from build123d import *

# Parameters (mm, degrees)
SKETCH1_W           = 315
SKETCH1_H           = 12.7
SKETCH1_W_2         = 50
BOSS_EXTRUDE1_DEPTH = 12.7
SKETCH2_R           = 3.75
CUT_EXTRUDE1_DEPTH  = 318.513983944


with BuildPart() as part:
    # Sketch1 → Boss-Extrude1 (new body)
    with BuildSketch(Plane(origin=(0, 0, 0), x_dir=(0, 0, -1), z_dir=(1, 0, 0))):
        with Locations((157.5, 6.35)):
            Rectangle(SKETCH1_W, SKETCH1_H)
        Polygon((15, 0), (0, 0), (0, -37.8), (15, -37.8), (15, -25.1), align=None)
        with Locations((40, -31.45)):
            Rectangle(SKETCH1_W_2, SKETCH1_H)
    extrude(amount=BOSS_EXTRUDE1_DEPTH)

    # Sketch2 → Cut-Extrude1 (cut, through all)
    with BuildSketch(Plane(origin=(12.7, 0, 0), x_dir=(0, 0, -1), z_dir=(1, 0, 0))):
        with Locations((7.5, 6.35)):
            Circle(SKETCH2_R)
        with Locations((207.5, 6.35)):
            Circle(SKETCH2_R)
    extrude(amount=-CUT_EXTRUDE1_DEPTH, mode=Mode.SUBTRACT)


solid = part.part
Read the model definition and answer for the solid it produces. Units are mm, in the model's axes. A direction names the side the tool comes from. Round coordinates to 2 decimals unless told otherwise and drop trailing zeros. Loops run counter-clockwise (first coordinate to the right, second up) from the corner with the lowest first, then second, coordinate; pieces in that order, holes last.
Q1. Section A-A on z = -207.5 is taken. Write down the section's boundary in (x, y), and give its area (3 significant figures).
Q2. Determine the mould class of faces 4 (the face through (6.439, 10.068, -7.012)), 5 (the face through (0, 1, -133)), 6 (the face through (6, 6, -315)) for opening direction Z: released by +Z, released by -Z, zero draft, split by the parting line, or undercut.
Q3. Section D-D on z = -7.5 is taken. Write down the section's boundary in (x, y).
Q4. Section B-B on x = 9 is taken. Write down the section's boundary in (y, z), and give its area (3 significant figures).
Q5. Which of the six approach directions +Z, -Z, +X, -X, +Y, -Y give full straight-line access (tool end or side, diameter ignored) to faces 1 (the face through (6, -32, -65)), 2 (the face through (6, -13, -15)), 3 (the face through (6, -12, 0))?
Q6. Section C-C on y = 6.35 is taken. Write down the section's boundary in (x, z).
Q7. Each of these flat-tipped pins is pushed along its axis until it touches: pin 1 (5 mm diameter, centred on x = 8, y = -23.5, fed in from +Z); pin 2 (6.5 mm diameter, centred on x = 6, y = -11, fed in from -Z); pin 3 (1 mm diameter, centred on y = -1.5, z = -265.5, fed in from -X); pin 4 (2 mm diameter, centred on x = 5, z = -229.5, fed in from -Y). Where does it stop, or does it pass through?
Q8. Consider probe 1 along Y at (x, z) = (5, -7.5); probe 2 along Z at (x, y) = (2, -22); probe 3 along Y at (x, z) = (5, -111). Determine where each line is inside the solid, lowest interval first.
Output:
1. outline: (0, 0) - (12.7, 0) - (12.7, 2.6) - (0, 2.6) - close; (0, 10.1) - (12.7, 10.1) - (12.7, 12.7) - (0, 12.7) - close
1. area: 66.0 mm2
2. face 4: undercut
2. face 5: zero draft
2. face 6: released by -Z
3. outline: (0, -37.8) - (12.7, -37.8) - (12.7, 2.6) - (0, 2.6) - close; (0, 10.1) - (12.7, 10.1) - (12.7, 12.7) - (0, 12.7) - close
4. outline: (-37.8, -65) - (-25.1, -65) - (-25.1, -15) - (0, -15) - (0, -315) - (12.7, -315) - (12.7, 0) - (-37.8, 0) - close; hole circle Ø7.5 at (6.35, -207.5); hole circle Ø7.5 at (6.35, -7.5)
4. area: 5,110 mm2
5. face 1: -Z, +X, -X, -Y
5. face 2: -Z, +X, -X
5. face 3: +Z, +X, -X, +Y, -Y
6. outline: (0, -315) - (12.7, -315) - (12.7, -211.25) - (0, -211.25) - close; (0, -203.75) - (12.7, -203.75) - (12.7, -11.25) - (0, -11.25) - close; (0, -3.75) - (12.7, -3.75) - (12.7, 0) - (0, 0) - close
7. pin 1: stops at z = 0
7. pin 2: stops at z = -15
7. pin 3: passes through
7. pin 4: stops at y = 0
8. probe 1: y = -37.8 to 2.6, 10.1 to 12.7
8. probe 2: z = -15 to 0
8. probe 3: y = 0 to 12.7
